from build123d import *

# Parameters (mm, degrees)
F0_R     = 20
F0_R_2   = 5
F1_DEPTH = 7.5
F3_R     = 7.5
F4_DEPTH = 131.4595038823
F5_W     = 100
F5_H     = 50
F6_DEPTH = 3
F7_R     = 4
F8_DEPTH = 3


with BuildPart() as f1:
    # F0 (on Front) → F1 (new body, symmetric)
    with BuildSketch(Plane.XZ):
        Circle(F0_R)
        Circle(F0_R_2, mode=Mode.SUBTRACT)
    extrude(amount=F1_DEPTH, both=True)

    # F3 (on offset) → F4 (join, through all)
    with BuildSketch(Plane.YZ.offset(150)):
        Circle(F3_R)
    extrude(amount=-F4_DEPTH)

    # F5 (on offset) → F6 (join)
    with BuildSketch(Plane.YZ.offset(150)):
        Rectangle(F5_W, F5_H)
    extrude(amount=F6_DEPTH)

    # F7 (on face) → F8 (cut, through all)
    with BuildSketch(Plane.YZ.offset(153)):
        with Locations((-25, 0)):
            Circle(F7_R)
        with Locations((25, 0)):
            Circle(F7_R)
    extrude(amount=-F8_DEPTH, mode=Mode.SUBTRACT)


solid = f1.part
Work out the finished part from the listing and answer in its coordinate system (mm). A direction names the side the tool comes from. Coordinates: 2 decimals unless noted, no trailing zeros. Loops run counter-clockwise (first coordinate to the right, second up) from the corner with the lowest first, then second, coordinate; pieces in that order, holes last. Notation, with made-up numbers: M 42.5,68 L 46.5,68 A37 cw 46.5,105 Z; hole C 4.25,42 d4. An arc over 180 degrees is marked long. Answer in a Markdown table with one row per item. Add a question column.
1. A tool of negligible diameter and unlimited length cuts with its end or side. For faces 1 (the flat face through (4, 7.5, -4)), 2 (the cylindrical face through (85.19, -7.493, 0.33)), 3 (the flat face through (153, -1, 0)), from which of +Z, -Z, +X, -X, +Y, -Y can it reach the whole face along a straight path? Write none if from no direction.
2. Flat-ended cylindrical pins translate along their axes: P1, Ø9, axis at x = 0, z = 0, coming from the +Y side; P2, Ø10, axis at y = -31.5, z = -4.5, coming from the -X side; P3, Ø8, axis at x = 123.5, z = 2, coming from the +Y side; P4, Ø25, axis at y = 15.5, z = -1, coming from the -X side. Find the tip coordinate at first contact, or state that the pin passes through.
3. The mould has two halves that part along Y. Classify faces 4 (the cylindrical face through (151.5, 21.8, -2.4)), 5 (the cylindrical face through (-1.08, 0.11, -4.88)), 6 (the flat face through (4, -7.5, -4)): pulls with the +Y half, pulls with the -Y half, needs draft (parallel to the pull), parting line crosses it, or undercut.
4. Find section C-C, the plane z = 2. Write down the section's boundary in (x, y), then the cut area to 3 significant figures.
5. Consider L1, parallel to Z at x = 0, y = 3.25; L2, parallel to Z at x = 151.5, y = -25; L3, parallel to X at y = 36, z = -1. Determine where each line is inside the solid, lowest interval first.
6. Find section A-A, the plane x = 0. Write down the section's boundary in (y, z), then the cut area to 3 significant figures.
7. Find section B-B, the plane y = -3. Write down the section's boundary in (x, z).
8. Find section D-D, the plane x = 39. Write down the section's boundary in (y, z), then the cut area to 3 significant figures.
Reported:
| question | item | result |
|---|---|---|
| 1 | face 1 | +Z, -Z, -X, +Y |
| 1 | face 2 | none |
| 1 | face 3 | +Z, -Z, +X, +Y, -Y |
| 2 | P1 | passes through |
| 2 | P2 | stops at x = 150 |
| 2 | P3 | stops at y = 7.5 |
| 2 | P4 | stops at x = -20 |
| 3 | face 4 | undercut |
| 3 | face 5 | needs draft |
| 3 | face 6 | pulls with the -Y half |
| 4 | outline | M -19.9,-7.5 L -4.58,-7.5 L -4.58,7.5 L -19.9,7.5 Z; M 4.58,-7.5 L 19.9,-7.5 L 19.9,-7.23 L 150,-7.23 L 150,-21.54 L 153,-21.54 L 153,21.54 L 150,21.54 L 150,7.23 L 19.9,7.23 L 19.9,7.5 L 4.58,7.5 Z; M 150,-50 L 153,-50 L 153,-28.46 L 150,-28.46 Z; M 150,28.46 L 153,28.46 L 153,50 L 150,50 Z |
| 4 | area | 2,600 mm^2 |
| 5 | L1 | z = -20 to -5, 5 to 20 |
| 5 | L2 | z = -25 to -4, 4 to 25 |
| 5 | L3 | x = 150 to 153 |
| 6 | outline | M -7.5,-20 L 7.5,-20 L 7.5,-5 L -7.5,-5 Z; M -7.5,5 L 7.5,5 L 7.5,20 L -7.5,20 Z |
| 6 | area | 450 mm^2 |
| 7 | outline | M 18.78,-6.87 L 150,-6.87 L 150,-25 L 153,-25 L 153,25 L 150,25 L 150,6.87 L 18.78,6.87 A20 ccw long Z; hole C 0,0 d10 |
| 8 | outline | C 0,0 d15 |
| 8 | area | 177 mm^2 |
